Input: part model. Units: mm. Frame: model coordinates. A direction names the side the tool comes from. Give positions to 0.01 mm unless a question says otherwise; leave off trailing zeros. Order: outer loops, then holes, each group sorted by start corner. A loop starts at its lowest first (then second) coordinate and runs counter-clockwise, first axis right, second up. Notation, with made-up numbers: (83.25, 75.5) - (139.25, 75.5) arc R19 cw to (139.25, 86.5) - close; hole circle Ø10 at (57, 15). An arc over 180 degrees is marked (long way). Answer in a Markdown table with one row per item. Add a question column.
1. Section query A-A on y = 7.25. Count the separate pieces of the cut face and the enclosed holes in it, and give its area (3 significant figures).
2. Section query B-B on z = -286. Return loops of the section in (x, y).
3. Contact query for flat-ended pins moving along their axis: pin 1 (6 mm diameter, centred on x = 195.5, y = 5, fed in from -Z); pin 2 (3 mm diameter, centred on x = -86, z = -285, fed in from -Y); pin 3 (10 mm diameter, centred on x = -209, z = -76, fed in from -Y); pin 4 (1.5 mm diameter, centred on y = 4, z = -84.5, fed in from -X). Output: stop coordinate, or through.
4. Ray query, line 1 (Y direction, x = 150, z = -152); line 2 (Y direction, x = -55, z = -67). Return the intervals inside material, ascending. Write a range as [from, to].
5. Access query for faces 1 (the face through (3.78, 5.24, -312.5)), 2 (the face through (3.78, 4.757, -285.725)). Directions: +Z, -Z, +X, -X, +Y, -Y. A direction counts if a zero-diameter tool reaches every point of the face in a straight line with its end or side. Return the directions, or none.
```python
from build123d import *

# Parameters (mm, degrees)
SKETCH2_W           = 540
SKETCH2_H           = 10
BOSS_EXTRUDE1_DEPTH = 3
EXTRUDE_THIN1_DEPTH = 540


with BuildPart() as part:
    # Sketch2 → Boss-Extrude1 (new body)
    with BuildSketch(Plane.XY):
        with Locations((0, 5)):
            Rectangle(SKETCH2_W, SKETCH2_H)
    extrude(amount=BOSS_EXTRUDE1_DEPTH)

    # Sketch3 → Extrude-Thin1 (add, through all)
    with BuildSketch(Plane(origin=(270, 0, 0), x_dir=(0, 0, -1), z_dir=(1, 0, 0))):
        Polygon((0.150284541, -0.199786278), (13.293867572, 9.687165702), (26.587735145, -0.312834298), (39.881602717, 9.687165702), (53.175470289, -0.312834298), (66.469337861, 9.687165702), (79.763205434, -0.312834298), (93.057073006, 9.687165702), (106.350940578, -0.312834298), (119.64480815, 9.687165702), (132.938675723, -0.312834298), (146.232543295, 9.687165702), (159.526410867, -0.312834298), (172.820278439, 9.687165702), (186.114146012, -0.312834298), (199.408013584, 9.687165702), (212.701881156, -0.312834298), (225.995748728, 9.687165702), (239.289616301, -0.312834298), (252.583483873, 9.687165702), (265.877351445, -0.312834298), (279.171219017, 9.687165702), (292.46508659, -0.312834298), (305.758954162, 9.687165702), (319.052821734, -0.312834298), (332.346689306, 9.687165702), (345.490272338, -0.199786278), (345.790841419, 0.199786278), (332.346689306, 10.312834298), (319.052821734, 0.312834298), (305.758954162, 10.312834298), (292.46508659, 0.312834298), (279.171219017, 10.312834298), (265.877351445, 0.312834298), (252.583483873, 10.312834298), (239.289616301, 0.312834298), (225.995748728, 10.312834298), (212.701881156, 0.312834298), (199.408013584, 10.312834298), (186.114146012, 0.312834298), (172.820278439, 10.312834298), (159.526410867, 0.312834298), (146.232543295, 10.312834298), (132.938675723, 0.312834298), (119.64480815, 10.312834298), (106.350940578, 0.312834298), (93.057073006, 10.312834298), (79.763205434, 0.312834298), (66.469337861, 10.312834298), (53.175470289, 0.312834298), (39.881602717, 10.312834298), (26.587735145, 0.312834298), (13.293867572, 10.312834298), (-0.150284541, 0.199786278), align=None)
    extrude(amount=-EXTRUDE_THIN1_DEPTH)


solid = part.part
```
Answer:
| question | item | result |
|---|---|---|
| 1 | separate pieces | 27 |
| 1 | enclosed holes | 0 |
| 1 | area | 13,300 mm² |
| 2 | outline | (-270, 4.55) - (270, 4.55) - (270, 5.18) - (-270, 5.18) - close |
| 3 | pin 1 | stops at z = -343.4 |
| 3 | pin 2 | stops at y = 4.17 |
| 3 | pin 3 | stops at y = -0.31 |
| 3 | pin 4 | stops at x = -270 |
| 4 | line 1 | y = [5.35, 5.97] |
| 4 | line 2 | y = [9.29, 9.91] |
| 5 | face 1 | +X, -X, +Y |
| 5 | face 2 | +X, -X, -Y |
